Geometry check sheet. Reference: the model listing, model coordinates, mm. Face numbers are marked on the shaded views. A direction names the side the tool comes from. Coordinates: 2 decimals unless noted, no trailing zeros. Write each loop counter-clockwise with the first axis right and the second up, starting at its lowest first coordinate (ties: lowest second). Pieces come first, ordered by that corner, then holes. Notation, with made-up numbers: (44.5, -9.75) -> (75.5, -9.75) arc R10 ccw to (75.5, -3.75) -> close; hole circle Ø1 at (-5, -38.75). An arc over 180 degrees is marked (long way). Answer in a Markdown table with one row per item. Add a question column.
Q1. Tool access check on the marked faces 5, 6 and 7. Record the directions out of +Z, -Z, +X, -X, +Y, -Y that give a thin tool (end or side, any length) a straight path to the whole face; none if there is none.
Q2. Thickness scan on line 1 (X direction, y = 11.75, z = 0); line 2 (X direction, y = 4.75, z = 0); line 3 (Z direction, x = -2.5, y = 18.25). Record the ranges inside material, lowest first.
Q3. Section check A-A, the plane y = 12. Record the boundary of the cut face in (x, z).
Q4. Release check for a two-part mould opening along X. For the marked faces 1, 2, 3 and 4 record: pulls with the +X half, pulls with the -X half, needs draft (parallel to the pull), parting line crosses it, or undercut.
Q5. Section check B-B, the plane y = 5.5. Record the boundary of the cut face in (x, z).
Q6. Gauge pin test, flat ends, axial feed: P1, Ø1.6, axis at x = 2.5, z = -0.5, coming from the -Y side; P2, Ø1.6, axis at y = 13, z = 0, coming from the -X side; P3, Ø2.5, axis at x = -1, z = 0, coming from the -Y side. Record the tip position at first contact, or that the pin passes through.
```python
from build123d import *

# Parameters (mm, degrees)
SKETCH1_R               = 12.75
BOSS_EXTRUDE1_DEPTH     = 20
CUT_EXTRUDE1_DEPTH      = 27.928145127
CUT_EXTRUDE1_DEPTH_BACK = 18.3
SKETCH2_R               = 3.05
SKETCH3_R               = 3.5
CUT_EXTRUDE2_DEPTH      = 6
FILLET1_R               = 3
SKETCH5_R               = 4
CUT_EXTRUDE3_DEPTH      = 14
FILLET3_R               = 3
BOSS_EXTRUDE2_START     = 10
BOSS_EXTRUDE2_DEPTH     = 10


with BuildPart() as part:
    # Sketch1 → Boss-Extrude1 (new body)
    with BuildSketch(Plane(origin=(0, 0, 0), x_dir=(1, 0, 0), z_dir=(0, 1, 0))):
        with Locations(Location((0, 0, 0), (0, 0, 270))):
            Circle(SKETCH1_R)
    extrude(amount=BOSS_EXTRUDE1_DEPTH)

    # Sketch2 → Cut-Extrude1 (cut, two sides: drawn at the far end of the back side and taken through both)
    with BuildSketch(Plane.XZ.offset(-CUT_EXTRUDE1_DEPTH_BACK)):
        with Locations(Location((0, 0, 0), (0, 0, 90))):
            Circle(SKETCH2_R)
    extrude(amount=CUT_EXTRUDE1_DEPTH + CUT_EXTRUDE1_DEPTH_BACK, mode=Mode.SUBTRACT)

    # Sketch3 → Cut-Extrude2 (cut)
    with BuildSketch(Plane.XZ):
        with Locations(Location((0, 0, 0), (0, 0, 270))):
            Circle(SKETCH3_R)
    extrude(amount=-CUT_EXTRUDE2_DEPTH, mode=Mode.SUBTRACT)

    # Fillet1
    fillet1_edges = [part.edges().sort_by_distance(p)[0] for p in [
        (0, 20, -12.75),
    ]]
    fillet(fillet1_edges, radius=FILLET1_R)

    # Sketch5 → Cut-Extrude3 (cut)
    with BuildSketch(Plane(origin=(0, 20, 0), x_dir=(1, 0, 0), z_dir=(0, 1, 0))):
        with Locations((0, 15.5)):
            Circle(SKETCH5_R)
        with Locations((10.960155108, 10.960155108)):
            Circle(SKETCH5_R)
        with Locations((15.5, 0)):
            Circle(SKETCH5_R)
        with Locations((10.960155108, -10.960155108)):
            Circle(SKETCH5_R)
        with Locations((0, -15.5)):
            Circle(SKETCH5_R)
        with Locations((-10.960155108, -10.960155108)):
            Circle(SKETCH5_R)
        with Locations((-15.5, 0)):
            Circle(SKETCH5_R)
        with Locations((-10.960155108, 10.960155108)):
            Circle(SKETCH5_R)
    extrude(amount=-CUT_EXTRUDE3_DEPTH, mode=Mode.SUBTRACT)

    # Fillet3
    # the kernel refuses this fillet: 3 mm, written as the material it adds along each edge
    with BuildSketch(Plane(origin=(0, 6, 15.5), x_dir=(0.5240999982324142, 0, 0.8516567335803691), z_dir=(-0.8516567335803691, 0, 0.5240999982324142))) as fillet3_piece_1_section:
        with BuildLine():
            CenterArc((4 - FILLET3_R, FILLET3_R), FILLET3_R, 270, 90)
            Line((4 - FILLET3_R, 0), (4, 0))
            Line((4, 0), (4, FILLET3_R))
        make_face()
    fillet3_piece_1 = revolve(axis=Axis((0, 6, 15.5), (0, 1, 0)), revolution_arc=296.784649365, mode=Mode.PRIVATE)
    fillet3_piece_1 = fillet3_piece_1 & Plane(origin=(0, 6.906503108, 0), x_dir=(0, 0, 1), z_dir=(0, -1, 0)) * Cylinder(12.75, 17, mode=Mode.PRIVATE)
    add(fillet3_piece_1)
    with BuildSketch(Plane(origin=(-10.960155108, 6, 10.960155108), x_dir=(-0.2316175887878651, 0, 0.9728069143278617), z_dir=(-0.9728069143278617, 0, -0.2316175887878651))) as fillet3_piece_2_section:
        with BuildLine():
            CenterArc((4 - FILLET3_R, FILLET3_R), FILLET3_R, 270, 90)
            Line((4, FILLET3_R), (4, 0))
            Line((4, 0), (4 - FILLET3_R, 0))
        make_face()
    fillet3_piece_2 = revolve(axis=Axis((-10.960155108, 6, 10.960155108), (0, 1, 0)), revolution_arc=296.784649365, mode=Mode.PRIVATE)
    fillet3_piece_2 = fillet3_piece_2 & Plane(origin=(0, 6.906501973, 0), x_dir=(0, 0, 1), z_dir=(0, -1, 0)) * Cylinder(12.75, 16, mode=Mode.PRIVATE)
    add(fillet3_piece_2)
    with BuildSketch(Plane(origin=(-15.5, 6, 0), x_dir=(-0.8516567335803689, 0, -0.524099998232414), z_dir=(-0.524099998232414, 0, 0.8516567335803689))) as fillet3_piece_3_section:
        with BuildLine():
            CenterArc((4 - FILLET3_R, -FILLET3_R), FILLET3_R, 0, 90)
            Line((4, -FILLET3_R), (4, 0))
            Line((4, 0), (4 - FILLET3_R, 0))
        make_face()
    fillet3_piece_3 = revolve(axis=Axis((-15.5, 6, 0), (0, -1, 0)), revolution_arc=296.784649365, mode=Mode.PRIVATE)
    fillet3_piece_3 = fillet3_piece_3 & Plane(origin=(0, 6.90650195, 0), x_dir=(0, 0, 1), z_dir=(0, -1, 0)) * Cylinder(12.75, 16, mode=Mode.PRIVATE)
    add(fillet3_piece_3)
    with BuildSketch(Plane(origin=(-10.960155108, 6, -10.960155108), x_dir=(-0.9728069143278615, 0, -0.23161758878786548), z_dir=(0.23161758878786548, 0, -0.9728069143278615))) as fillet3_piece_4_section:
        with BuildLine():
            CenterArc((4 - FILLET3_R, FILLET3_R), FILLET3_R, 270, 90)
            Line((4, FILLET3_R), (4, 0))
            Line((4, 0), (4 - FILLET3_R, 0))
        make_face()
    fillet3_piece_4 = revolve(axis=Axis((-10.960155108, 6, -10.960155108), (0, 1, 0)), revolution_arc=296.784649365, mode=Mode.PRIVATE)
    fillet3_piece_4 = fillet3_piece_4 & Plane(origin=(0, 6.906501973, 0), x_dir=(0, 0, 1), z_dir=(0, -1, 0)) * Cylinder(12.75, 17, mode=Mode.PRIVATE)
    add(fillet3_piece_4)
    with BuildSketch(Plane(origin=(0, 6, -15.5), x_dir=(-0.5240999982324135, 0, -0.8516567335803694), z_dir=(0.8516567335803694, 0, -0.5240999982324135))) as fillet3_piece_5_section:
        with BuildLine():
            CenterArc((4 - FILLET3_R, FILLET3_R), FILLET3_R, 270, 90)
            Line((4, FILLET3_R), (4, 0))
            Line((4, 0), (4 - FILLET3_R, 0))
        make_face()
    fillet3_piece_5 = revolve(axis=Axis((0, 6, -15.5), (0, 1, 0)), revolution_arc=296.784649365, mode=Mode.PRIVATE)
    fillet3_piece_5 = fillet3_piece_5 & Plane(origin=(0, 6.906501973, 0), x_dir=(0, 0, 1), z_dir=(0, -1, 0)) * Cylinder(12.75, 16, mode=Mode.PRIVATE)
    add(fillet3_piece_5)
    with BuildSketch(Plane(origin=(10.960155108, 6, -10.960155108), x_dir=(0.2316175887878651, 0, -0.9728069143278617), z_dir=(0.9728069143278617, 0, 0.2316175887878651))) as fillet3_piece_6_section:
        with BuildLine():
            CenterArc((4 - FILLET3_R, FILLET3_R), FILLET3_R, 270, 90)
            Line((4, FILLET3_R), (4, 0))
            Line((4, 0), (4 - FILLET3_R, 0))
        make_face()
    fillet3_piece_6 = revolve(axis=Axis((10.960155108, 6, -10.960155108), (0, 1, 0)), revolution_arc=296.784649365, mode=Mode.PRIVATE)
    fillet3_piece_6 = fillet3_piece_6 & Plane(origin=(0, 6.906501973, 0), x_dir=(0, 0, 1), z_dir=(0, -1, 0)) * Cylinder(12.75, 16, mode=Mode.PRIVATE)
    add(fillet3_piece_6)
    with BuildSketch(Plane(origin=(15.5, 6, 0), x_dir=(0.8516567335803694, 0, -0.5240999982324135), z_dir=(0.5240999982324135, 0, 0.8516567335803694))) as fillet3_piece_7_section:
        with BuildLine():
            CenterArc((4 - FILLET3_R, FILLET3_R), FILLET3_R, 270, 90)
            Line((4, FILLET3_R), (4, 0))
            Line((4, 0), (4 - FILLET3_R, 0))
        make_face()
    fillet3_piece_7 = revolve(axis=Axis((15.5, 6, 0), (0, 1, 0)), revolution_arc=296.784649365, mode=Mode.PRIVATE)
    fillet3_piece_7 = fillet3_piece_7 & Plane(origin=(0, 6.906501973, 0), x_dir=(0, 0, 1), z_dir=(0, -1, 0)) * Cylinder(12.75, 17, mode=Mode.PRIVATE)
    add(fillet3_piece_7)
    with BuildSketch(Plane(origin=(10.960155108, 6, 10.960155108), x_dir=(0.9728069143278617, 0, 0.2316175887878651), z_dir=(-0.2316175887878651, 0, 0.9728069143278617))) as fillet3_piece_8_section:
        with BuildLine():
            CenterArc((4 - FILLET3_R, FILLET3_R), FILLET3_R, 270, 90)
            Line((4, FILLET3_R), (4, 0))
            Line((4, 0), (4 - FILLET3_R, 0))
        make_face()
    fillet3_piece_8 = revolve(axis=Axis((10.960155108, 6, 10.960155108), (0, 1, 0)), revolution_arc=296.784649365, mode=Mode.PRIVATE)
    fillet3_piece_8 = fillet3_piece_8 & Plane(origin=(0, 6.906501973, 0), x_dir=(0, 0, 1), z_dir=(0, -1, 0)) * Cylinder(12.75, 16, mode=Mode.PRIVATE)
    add(fillet3_piece_8)

    # Sketch6 → Boss-Extrude2 (add)
    with BuildSketch(Plane.XZ.offset(-18.3).offset(BOSS_EXTRUDE2_START)):
        with BuildLine():
            Line((1.6, 2.596632435), (1.6, -2.596632435))
            ThreePointArc((1.6, -2.596632435), (3.05, 0), (1.6, 2.596632435))
        make_face()
    extrude(amount=-BOSS_EXTRUDE2_DEPTH)


solid = part.part
```
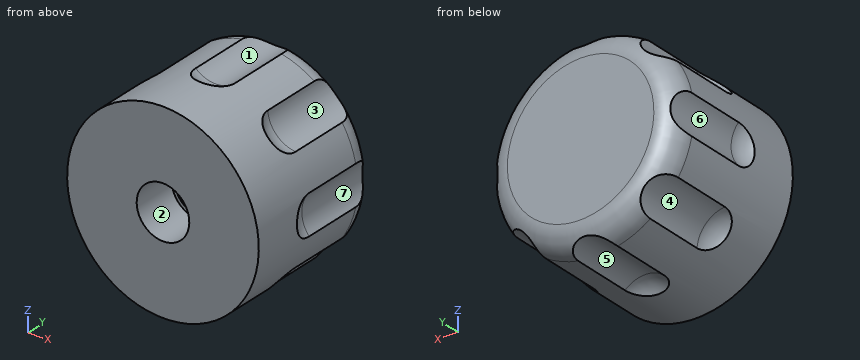
Calculated:
| question | item | result |
|---|---|---|
| 1 | face 5 | -Z, +Y |
| 1 | face 6 | -X, +Y |
| 1 | face 7 | +X, +Y |
| 2 | line 1 | x = -11.5 to -3.05, 1.6 to 11.5 |
| 2 | line 2 | x = -12.75 to -3.5, 3.5 to 12.75 |
| 2 | line 3 | z = -12.22 to -1.75, 1.75 to 12.22 |
| 3 | outline | (-12.48, -2.62) arc R12.75 ccw to (-10.68, -6.97) arc R4 cw to (-6.97, -10.68) arc R12.75 ccw to (-2.62, -12.48) arc R4 cw to (2.62, -12.48) arc R12.75 ccw to (6.97, -10.68) arc R4 cw to (10.68, -6.97) arc R12.75 ccw to (12.48, -2.62) arc R4 cw to (12.48, 2.62) arc R12.75 ccw to (10.68, 6.97) arc R4 cw to (6.97, 10.68) arc R12.75 ccw to (2.62, 12.48) arc R4 cw to (-2.62, 12.48) arc R12.75 ccw to (-6.97, 10.68) arc R4 cw to (-10.68, 6.97) arc R12.75 ccw to (-12.48, 2.62) arc R4 cw to start; hole (1.6, -2.6) -> (1.6, 2.6) arc R3.05 ccw (long way) to start |
| 4 | face 1 | undercut |
| 4 | face 2 | undercut |
| 4 | face 3 | pulls with the +X half |
| 4 | face 4 | pulls with the -X half |
| 5 | outline | circle Ø25.5 at (0, 0); hole circle Ø7 at (0, 0) |
| 6 | P1 | stops at y = 6 |
| 6 | P2 | stops at x = -11.58 |
| 6 | P3 | stops at y = 18.3 |
